```python
from build123d import *

# Parameters (mm, degrees)
SKETCH_1_R        = 8
SKETCH_1_R_2      = 4
EXTRUDE_1_DEPTH   = 10
EXTRUDE_1_2_DEPTH = 10
EXTRUDE_START     = 1
EXTRUDE_2_DEPTH   = 8
EXTRUDE_START_2   = -1
EXTRUDE_3_DEPTH   = 8
SKETCH_5_R        = 8
SKETCH_5_R_2      = 4
EXTRUDE_4_DEPTH   = 10


with BuildPart() as part:
    # Sketch 1 → Extrude 1 (new body)
    with BuildSketch(Plane.XY):
        Circle(SKETCH_1_R)
        Circle(SKETCH_1_R_2, mode=Mode.SUBTRACT)
    extrude(amount=EXTRUDE_1_DEPTH)



with BuildPart() as body_2:
    # Sketch 1 → Extrude 1 2 (new body)
    with BuildSketch(Plane.XY):
        with Locations((-53.605968084, 26.951812291)):
            Circle(SKETCH_1_R)
        with Locations((-53.605968084, 26.951812291)):
            Circle(SKETCH_1_R_2, mode=Mode.SUBTRACT)
    extrude(amount=EXTRUDE_1_2_DEPTH)


with BuildPart() as part_1:
    add(part.part)

    add(body_2.part)  # Extrude 2 merges body 2
    # Sketch 3 → Extrude 2 (add)
    with BuildSketch(Plane.XY.offset(EXTRUDE_START)):
        with BuildLine():
            Line((-51.573547302, 19.214289059), (-7.42278324, -2.983670385))
            ThreePointArc((-7.42278324, -2.983670385), (-7.147462411, 3.593574972), (-2.032420782, 7.737523232))
            Line((-2.032420782, 7.737523232), (-46.183184844, 29.935482676))
            ThreePointArc((-46.183184844, 29.935482676), (-46.458505673, 23.358237319), (-51.573547302, 19.214289059))
        make_face()
    extrude(amount=EXTRUDE_2_DEPTH)



with BuildPart() as body_2_2:
    # Sketch 4 → Extrude 3 (new body)
    with BuildSketch(Plane.XY.offset(EXTRUDE_START_2)):
        with BuildLine():
            Line((6.92820323, 4), (26.92820323, -30.641016151))
            ThreePointArc((26.92820323, -30.641016151), (33.036798625, -45.545943872), (34.959960983, -61.538856509))
            ThreePointArc((34.959960983, -61.538856509), (41.911210079, -98.657642521), (62.774179905, -130.135581289))
            ThreePointArc((62.774179905, -130.135581289), (62.827441336, -138.566924041), (54.397444356, -138.726699833))
            ThreePointArc((54.397444356, -138.726699833), (26.885397662, -101.001387411), (14.477282647, -55.988604867))
            ThreePointArc((14.477282647, -55.988604867), (11.073298234, -38.952300047), (4.07179677, -23.052558883))
            Line((4.07179677, -23.052558883), (-6.92820323, -4))
            ThreePointArc((-6.92820323, -4), (4, -6.92820323), (6.92820323, 4))
        make_face()
    extrude(amount=-EXTRUDE_3_DEPTH)


with BuildPart() as part_2:
    add(part_1.part)

    add(body_2_2.part)  # Extrude 4 merges body 2 2
    # Sketch 5 → Extrude 4 (add)
    with BuildSketch(Plane.XY):
        Circle(SKETCH_5_R)
        Circle(SKETCH_5_R_2, mode=Mode.SUBTRACT)
    extrude(amount=-EXTRUDE_4_DEPTH)


solid = part_2.part
```
Source: CAD feature listing. Evaluate the final solid. Frame: model axes, mm. Give positions to 0.01 mm unless a question says otherwise; leave off trailing zeros. Loops run counter-clockwise (first coordinate to the right, second up) from the corner with the lowest first, then second, coordinate; pieces in that order, holes last. Notation, with made-up numbers: (48.25, 67.25) - (88.25, 67.25) arc R21 ccw to (88.25, 98.25) - close; hole circle Ø6 at (56.5, 58.5). An arc over 180 degrees is marked (long way). Use CSV: the item, a comma, the result in double quotes. Start each with the question number.
1. Section D-D (z = 3.25). Output: boundary loops of the cut face in (x, y), then the cut area to 3 significant figures.
2. Draft query along Y for faces 1 (the cylindrical face through (-57.6, 27.13, 4.93)), 2 (the flat face through (-23.8, 18.68, 4.94)), 3 (the flat face through (-4, -2, -10)). Return one class per face: +Y half, -Y half, draft (parallel to the pull), parting line (faces both ways), or undercut.
3. Ray query, L1, parallel to Y at x = 0, z = 6.5; L2, parallel to Y at x = -53, z = 2.25; L3, parallel to Z at x = 30, y = -41. Return the intervals inside material, ascending.
4. Pin query (flat end, axial travel): pin 1 (12 mm diameter, centred on x = 11, y = 16, fed in from +Z) (3 decimals); pin 2 (1.5 mm diameter, centred on y = -8, z = 7, fed in from +X); pin 3 (1.5 mm diameter, centred on y = -4.5, z = -7.5, fed in from -X); pin 4 (5 mm diameter, centred on x = -51.5, y = 29.5, fed in from -Z). Return the tip coordinate at first contact, or that it passes through.
5. Section C-C (z = -5). Output: boundary loops of the cut face in (x, y), then the cut area to 3 significant figures.
6. Section A-A (x = 0). Output: boundary loops of the cut face in (y, z).
7. Section B-B (y = 0). Output: boundary loops of the cut face in (x, z).
Response:
1,outline,"(-51.57, 19.21) - (-7.42, -2.98) arc R8 ccw (long way) to (-2.03, 7.74) - (-46.18, 29.94) arc R8 ccw (long way) to start; hole circle Ø8 at (-53.61, 26.95); hole circle Ø8 at (0, 0)"
1,area,"850 mm²"
2,face 1,"undercut"
2,face 2,"+Y half"
2,face 3,"draft"
3,L1,"-8 to -4, 4 to 8"
3,L2,"18.97 to 23, 30.91 to 34.93"
3,L3,"-9 to -1"
4,pin 1,"through"
4,pin 2,"x = 3.38"
4,pin 3,"x = -7.07"
4,pin 4,"z = 0"
5,outline,"(-6.93, -4) - (4.07, -23.05) arc R80 cw to (14.48, -55.99) arc R130 ccw to (54.4, -138.73) arc R6 ccw to (62.77, -130.14) arc R95 cw to (34.96, -61.54) arc R60 ccw to (26.93, -30.64) - (6.93, 4) arc R8 ccw to start; hole circle Ø8 at (0, 0)"
5,area,"2,520 mm²"
6,outline,"(-16, -9) - (-8, -9) - (-8, -10) - (-4, -10) - (-4, 10) - (-8, 10) - (-8, -1) - (-16, -1) - close; (4, -10) - (8, -10) - (8, 10) - (4, 10) - close"
7,outline,"(-13.36, 1) - (-8, 1) - (-8, -10) - (-4, -10) - (-4, 10) - (-8, 10) - (-8, 9) - (-13.36, 9) - close; (4, -10) - (8, -10) - (8, -9) - (9.24, -9) - (9.24, -1) - (8, -1) - (8, 10) - (4, 10) - close"
